Check sheet for the modelled part. Datum: model origin and axes. Units: mm. A direction names the side the tool comes from. Round coordinates to 2 decimals unless told otherwise and drop trailing zeros. Write each loop counter-clockwise with the first axis right and the second up, starting at its lowest first coordinate (ties: lowest second). Pieces come first, ordered by that corner, then holes. Notation, with made-up numbers: (0.5, 65) - (42.5, 65) arc R23 ccw to (42.5, 77) - close; hole circle Ø3 at (37, -3). An arc over 180 degrees is marked (long way). Answer as a JSON object with one key per item and string values. Group by question number.
Item 1: Gauge pin test, flat ends, axial feed: P1, Ø1.1, axis at y = -3, z = 40, coming from the +X side; P2, Ø4.5, axis at x = -5, y = 2, coming from the -Z side; P3, Ø2, axis at x = -13, y = 4.5, coming from the +Z side. Record the tip position at first contact, or that the pin passes through.
Item 2: Sectioned sample at C-C on z = 27. Record the boundary of the cut face in (x, y), plus the area to 3 significant figures.
Item 3: Set-up check for faces 4 (the cylindrical face through (15.03, -0.38, 93.79)), 5 (the flat face through (-21, 0, 85)), 6 (the cylindrical face through (0.1, 2.9, 34.5)): record each of +Z, -Z, +X, -X, +Y, -Y from which the full face is reachable in a straight line by a thin tool's end or side.
Item 4: Sectioned sample at B-B on x = 4. Record the boundary of the cut face in (y, z), plus the area to 3 significant figures.
Item 5: Release check for a two-part mould opening along X. For faces 1 (the flat face through (-4, 0, 75)), 2 (the flat face through (-4, -7.5, 72)), 3 (the cylindrical face through (-23.859, 0.105, 71.203)) record: pulls with the +X half, pulls with the -X half, needs draft (parallel to the pull), parting line crosses it, or undercut.
Item 6: Thickness scan on line 1 (X direction, y = 1.25, z = 92); line 2 (Z direction, x = -17, y = -3); line 3 (Z direction, x = -23.9, y = 0) (3 decimals). Record the ranges inside material, lowest first.
Item 7: Sectioned sample at A-A on y = 6.25. Record the boundary of the cut face in (x, z).
```python
from build123d import *

# Parameters (mm, degrees)
F0_R      = 2.9
F1_DEPTH  = 70
F2_W      = 42
F2_H      = 15
F3_DEPTH  = 5
F4_W      = 4
F4_H      = 15
F5_DEPTH  = 25
F6_R      = 1.75
F7_DEPTH  = 50
F8_R      = 4
F10_DEPTH = 70


with BuildPart() as f1:
    # F0 (on Top) → F1 (new body)
    with BuildSketch(Plane.XY):
        Circle(F0_R)
    extrude(amount=F1_DEPTH)

    # F2 (on face) → F3 (join)
    with BuildSketch(Plane.XY.offset(70)):
        with Locations((-4, 0)):
            Rectangle(F2_W, F2_H)
    extrude(amount=F3_DEPTH)

    # F4 (on face) → F5 (join)
    with BuildSketch(Plane.XY.offset(75)):
        with Locations((-23, 0)):
            Rectangle(F4_W, F4_H)
        with Locations((15, 0)):
            Rectangle(F4_W, F4_H)
    extrude(amount=F5_DEPTH)

    # F6 (on face) → F7 (cut)
    with BuildSketch(Plane.YZ.offset(17)):
        with BuildLine():
            Line((-7.5, 75), (-4.45401, 96.141711))
            ThreePointArc((-4.45401, 96.141711), (-2.946379, 98.901301), (0, 100))
            Line((0, 100), (-7.5, 100))
            Line((-7.5, 100), (-7.5, 75))
        make_face()
        with Locations((0, 95.5)):
            Circle(F6_R)
        with BuildLine():
            Line((7.5, 100), (0, 100))
            ThreePointArc((0, 100), (2.946379, 98.901301), (4.45401, 96.141711))
            Line((4.45401, 96.141711), (7.5, 75))
            Line((7.5, 75), (7.5, 100))
        make_face()
    extrude(amount=-F7_DEPTH, mode=Mode.SUBTRACT)

    # F8
    f8_edges = [f1.edges().sort_by_distance(p)[0] for p in [
        (-25, 0, 70),
        (17, 0, 70),
    ]]
    fillet(f8_edges, radius=F8_R)

    # F9 (on face) → F10 (join)
    with BuildSketch(Plane(origin=(0, 0, 70), x_dir=(1, 0, 0), z_dir=(0, 0, -1))):
        with BuildLine():
            ThreePointArc((-0.5, 2.856571), (-1.865476, -2.22036), (2.9, 0))
            ThreePointArc((2.9, 0), (2.22036, 1.865476), (0.5, 2.856571))
            ThreePointArc((0.5, 2.856571), (0, 2.9), (-0.5, 2.856571))
        make_face()
        with BuildLine():
            ThreePointArc((-0.5, 2.856571), (0, 2.9), (0.5, 2.856571))
            Line((0.5, 2.856571), (0.5, 3.856571))
            Line((0.5, 3.856571), (-0.5, 3.856571))
            Line((-0.5, 3.856571), (-0.5, 2.856571))
        make_face()
    extrude(amount=F10_DEPTH)


solid = f1.part
```
Completed:
{
 "1": {"P1": "x = 1.55", "P2": "z = 70", "P3": "z = 75"},
 "2": {"outline": "(-0.5, -3.86) - (0.5, -3.86) - (0.5, -2.86) arc R2.9 ccw (long way) to (-0.5, -2.86) - close", "area": "27.4 mm²"},
 "3": {"face 4": "+X, -X", "face 5": "+Z, +Y, -Y", "face 6": "-Z"},
 "4": {"outline": "(-7.5, 70) - (7.5, 70) - (7.5, 75) - (-7.5, 75) - close", "area": "75.0 mm²"},
 "5": {"face 1": "undercut", "face 2": "needs draft", "face 3": "pulls with the -X half"},
 "6": {"line 1": "-25 to -21, 13 to 17", "line 2": "70 to 75", "line 3": "71.245 to 93.75, 97.25 to 100"},
 "7": {"outline": "(-25, 74) arc R4 ccw to (-21, 70) - (13, 70) arc R4 ccw to (17, 74) - (17, 83.68) - (13, 83.68) - (13, 75) - (-21, 75) - (-21, 83.68) - (-25, 83.68) - close"}
}
